The figure shows three views and two pictorial views of one solid part (mm, origin at its lowest corner). Answer the questions. A direction names the side the tool comes from. Coordinates: 2 decimals unless noted, no trailing zeros. Loops run counter-clockwise (first coordinate to the right, second up) from the corner with the lowest first, then second, coordinate; pieces in that order, holes last. Notation, with made-up numbers: (-14, 41) - (-6, 41) arc R19 cw to (-6, 66) - close; hole circle Ø8 at (46.5, 67.25). An arc over 180 degrees is marked (long way). Return JSON: item names as keys, results as strings. Group by question number.
1. The mould has two halves that part along X. Classify the marked faces 1, 2 and 3: pulls with the +X half, pulls with the -X half, needs draft (parallel to the pull), parting line crosses it, or undercut.
2. Each of these flat-tipped pins is pushed along its axis until it touches: P1, Ø1.4, axis at x = 12, z = 7.5, coming from the +Y side; P2, Ø1.5, axis at x = 6.5, z = 2, coming from the -Y side; P3, Ø1.5, axis at y = 19, z = 5, coming from the -X side (1 decimal). Where does it stop, or does it pass through?
3. Find the intervals of material crossed by line 1 along Y through (x, z) = (16, 5.5); line 2 along Y through (x, z) = (4.5, 5.25) (1 decimal); line 3 along X through (y, z) = (1.25, 3.25) (1 decimal), in increasing order.
4. Which of the six approach directions +Z, -Z, +X, -X, +Y, -Y give full straight-line access (tool end or side, diameter ignored) to the marked faces 4, 5 and 6?
5. Section B-B (z = 8.5) is taken. Write down the section's boundary in (x, y) (1 decimal).
6. Section C-C (z = 1) is taken. Write down the section's boundary in (x, y), and give its area (3 significant figures).
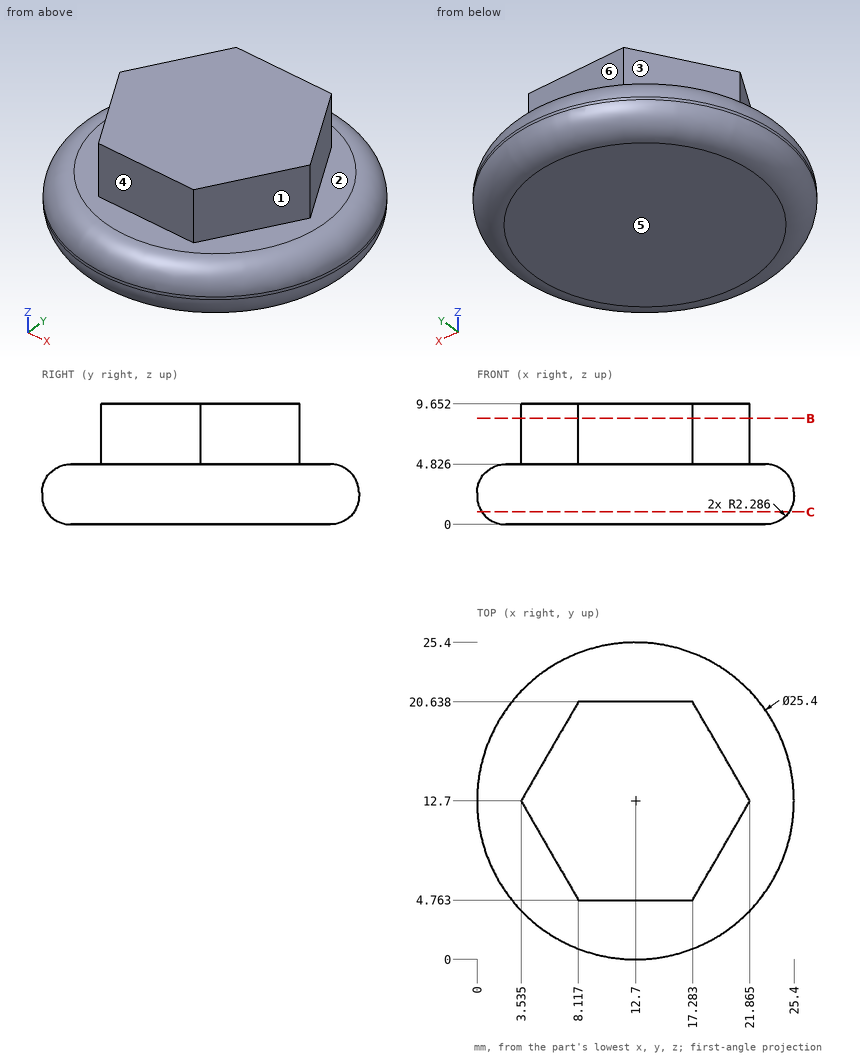
The answers:
{
 "1": {"face 1": "pulls with the +X half", "face 2": "needs draft", "face 3": "pulls with the -X half"},
 "2": {"P1": "stops at y = 20.64", "P2": "stops at y = 1.24", "P3": "stops at x = 2.5"},
 "3": {"line 1": "y = 4.76 to 20.64", "line 2": "y = 11 to 14.4", "line 3": "x = 7.5 to 17.9"},
 "4": {"face 4": "+Z, +X, -X, -Y", "face 5": "-Z, +X, -X, +Y, -Y", "face 6": "+Z, +X, -X, +Y"},
 "5": {"outline": "(3.5, 12.7) - (8.1, 4.8) - (17.3, 4.8) - (21.9, 12.7) - (17.3, 20.6) - (8.1, 20.6) - close"},
 "6": {"outline": "circle Ø24.61 at (12.7, 12.7)", "area": "476 mm2"}
}
